```python
from build123d import *

# Parameters (mm, degrees)
BOSS_EXTRUDE1_DEPTH = 31.75
SKETCH3_W           = 6.858
SKETCH3_H           = 6.35
SKETCH3_R           = 1.6383
CUT_EXTRUDE1_DEPTH  = 4.175
BOSS_EXTRUDE2_REACH = 21.05
SKETCH4_R           = 0.9525


with BuildPart() as part:
    # Sketch1 → Boss-Extrude1 (new body)
    with BuildSketch(Plane.XY):
        with BuildLine():
            Line((0, 0), (19.1262, 0))
            Line((19.1262, 0), (19.1262, 0.5588))
            Line((19.1262, 0.5588), (10.772204032, 0.5588))
            ThreePointArc((10.772204032, 0.5588), (9.5631, 3.175), (8.353995968, 0.5588))
            Line((8.353995968, 0.5588), (0, 0.5588))
            Line((0, 0.5588), (0, 0))
        make_face()
    extrude(amount=BOSS_EXTRUDE1_DEPTH)

    # Sketch3 → Cut-Extrude1 (cut, through all)
    with BuildSketch(Plane.XZ):
        with Locations((9.5631, 15.875)):
            Rectangle(SKETCH3_W, SKETCH3_H)
        with Locations((3.5814, 28.575)):
            Circle(SKETCH3_R)
        with Locations((15.5448, 28.575)):
            Circle(SKETCH3_R)
        with Locations((15.5448, 3.175)):
            Circle(SKETCH3_R)
        with Locations((3.5814, 3.175)):
            Circle(SKETCH3_R)
    extrude(amount=-CUT_EXTRUDE1_DEPTH, mode=Mode.SUBTRACT)

    # Sketch4 → Boss-Extrude2 (add, up to next)
    with BuildSketch(Plane.XY.offset(12.7), mode=Mode.PRIVATE) as boss_extrude2_sk1:
        with Locations((9.5631, 1.5875)):
            Circle(SKETCH4_R)
    boss_extrude2_tool1 = extrude(boss_extrude2_sk1.sketch, amount=BOSS_EXTRUDE2_REACH, mode=Mode.PRIVATE) - part.part
    add(boss_extrude2_tool1.solids().sort_by_distance((9.5631, 1.5875, 12.7))[0])


solid = part.part
```
Design review of the part built by this model. Coordinates are the model's own, in mm. A direction names the side the tool comes from. Give positions to 0.01 mm unless a question says otherwise; leave off trailing zeros. Order: outer loops, then holes, each group sorted by start corner. A loop starts at its lowest first (then second) coordinate and runs counter-clockwise, first axis right, second up. Notation, with made-up numbers: (-18, -24.75) -> (-9, -24.75) arc R32 cw to (-9, 13.25) -> close; hole circle Ø4 at (76, 35). An arc over 180 degrees is marked (long way). Write each question's results on one line, items separated by ' | '. Start each with the question number.
Q1. Machinability: for faces 4 (the flat face through (9, 0, 12)), 5 (the flat face through (10.3, 0.5, 12.7)), which of the approach directions +Z, -Z, +X, -X, +Y, -Y give a long, thin tool a straight path to every point of the face, cutting with its end or side? Answer none if there is none.
Q2. Add section B-B on z = 24.5. Give the boundary of the cut face in (x, y) (1 decimal).
Q3. Add section A-A on x = 3.75. Give the boundary of the cut face in (y, z), and give its area (3 significant figures).
Q4. For pin 1 (1.5 mm diameter, centred on x = 16, y = 1, fed in from +Z); pin 2 (4 mm diameter, centred on x = 4, z = 23, fed in from +Y); pin 3 (8 mm diameter, centred on x = 14.5, z = 23, fed in from +Y); pin 4 (2.5 mm diameter, centred on x = 3.58, z = 3.18, fed in from +Y), all flat-tipped, find the tip position at first contact; note any pin that passes through.
Q5. Add section C-C on z = 29. Give the boundary of the cut face in (x, y) (1 decimal).
Q6. Wall thickness on L1, parallel to Y at x = 14, z = 9.5; L2, parallel to Y at x = 9.5, z = 11; L3, parallel to Z at x = 4.25, y = 0.35: over which ranges is each line inside the solid? List them lowest first. Write a range as from..to.
Q7. Add section D-D on y = 1.1. Give the boundary of the cut face in (x, z), and give its area (3 significant figures).
Q8. Mouldability with a two-part tool opening along Z and no side actions: class faces 1 (the flat face through (4, 0.559, 16)), 2 (the cylindrical face through (15.33, 0.28, 30.2)), 3 (the flat face through (10, 1, 31.75)) as +Z half, -Z half, draft (parallel to the pull), parting line (faces both ways), or undercut.
Found:
1) face 4: +Z, -Z, +X, -X, -Y | face 5: none
2) outline: (0, 0) -> (19.1, 0) -> (19.1, 0.6) -> (10.8, 0.6) arc R1.6 ccw (long way) to (8.4, 0.6) -> (0, 0.6) -> close
3) outline: (0, 0) -> (0.56, 0) -> (0.56, 1.55) -> (0, 1.55) -> close; (0, 4.8) -> (0.56, 4.8) -> (0.56, 26.95) -> (0, 26.95) -> close; (0, 30.2) -> (0.56, 30.2) -> (0.56, 31.75) -> (0, 31.75) -> close | area: 14.1 mm2
4) pin 1: stops at z = 31.75 | pin 2: stops at y = 0.56 | pin 3: stops at y = 2.87 | pin 4: passes through
5) outline: (0, 0) -> (2, 0) -> (2, 0.6) -> (0, 0.6) -> close; (5.2, 0) -> (14, 0) -> (14, 0.6) -> (10.8, 0.6) arc R1.6 ccw (long way) to (8.4, 0.6) -> (5.2, 0.6) -> close; (17.1, 0) -> (19.1, 0) -> (19.1, 0.6) -> (17.1, 0.6) -> close
6) L1: y = 0..0.56 | L2: y = 0..3.17 | L3: z = 0..1.68, 4.67..27.08, 30.07..31.75
7) outline: (8.05, 0) -> (11.07, 0) -> (11.07, 12.7) -> (10.38, 12.7) -> (10.38, 19.05) -> (11.07, 19.05) -> (11.07, 31.75) -> (8.05, 31.75) -> (8.05, 19.05) -> (8.74, 19.05) -> (8.74, 12.7) -> (8.05, 12.7) -> close | area: 87.1 mm2
8) face 1: draft | face 2: undercut | face 3: +Z half
